Can you work these out from the model? Positions are in its coordinate system, mm. A direction names the side the tool comes from. Coordinates: 2 decimals unless noted, no trailing zeros. Order: outer loops, then holes, each group sorted by start corner. A loop starts at its lowest first (then second) coordinate and runs counter-clockwise, first axis right, second up. Notation, with made-up numbers: (-39, 30.25) - (16, 30.25) arc R22 cw to (16, 57.25) - close; hole circle Ø6 at (38, 74.5). An arc over 180 degrees is marked (long way). Return JSON: item names as keys, results as strings. Group by question number.
1) Which directions (+Z, -Z, +X, -X, +Y, -Y) give clear straight access to the entire face, cutting with the end or side of a thin tool? Please do faces 4 (the face through (2, -90.702, -6)), 5 (the face through (2, -103.702, -17)), 6 (the face through (1.97, -115.42, -86.6)).
2) For pin 1 Ø1 at (x, z) = (1, -129.5) entering from -Y; pin 2 Ø2 at (x, z) = (2.5, -23) entering from +Y; pin 3 Ø1.2 at (x, z) = (2.5, -37.5) entering from +Y, each with a flat end and sliding along its axis, tell me the tip position at first contact or that it passes through.
3) Imagine slicing it at A-A (y = -126). Write out the boundary of the cut face in (x, z) (3 decimals), and give its area (3 significant figures).
4) Imagine slicing it at D-D (y = -62.5). Write out the boundary of the cut face in (x, z).
5) If we mould it in two halves opening along Z, with no side actions, what happens to faces 1 (the face through (1.972, -92.206, 3.574)), 2 (the face through (2, -140.702, -33)), 3 (the face through (2, -130.702, -17))? For each: pulls with the +Z half, pulls with the -Z half, needs draft (parallel to the pull), parting line crosses it, or undercut.
6) Imagine slicing it at C-C (y = -113). Write out the boundary of the cut face in (x, z) (3 decimals), and give its area (3 significant figures).
7) If I drill on line 1 along Z through (x, y) = (2.2, -133) (3 decimals); line 2 along Z through (x, y) = (3.55, -105) (3 decimals); line 3 along Z through (x, y) = (3.1, -122) (3 decimals), over which ranges is the centre line in solid material (lowest first)?
```python
from build123d import *

# Parameters (mm, degrees)
SKETCH2_W           = 4
SKETCH2_H           = 27
BOSS_EXTRUDE1_DEPTH = 4
CUT_EXTRUDE1_DEPTH  = 10
BOSS_EXTRUDE2_DEPTH = 4


with BuildPart() as part:
    # Sketch2 → Boss-Extrude1 (new body)
    with BuildSketch(Plane(origin=(0, 0, 0), x_dir=(0, 0, -1), z_dir=(1, 0, 0))):
        with BuildLine():
            Line((53.344601804, -85.498776043), (74.987188297, -45.905868036))
            ThreePointArc((74.987188297, -45.905868036), (78.661054663, -42.101027368), (83.761812448, -40.70232204))
            Line((83.761812448, -40.70232204), (92.296503371, -40.70232204))
            Line((92.296503371, -40.70232204), (92.296503371, -44.70232204))
            Line((92.296503371, -44.70232204), (152.296503371, -44.70232204))
            Line((152.296503371, -44.70232204), (152.296503371, -40.70232204))
            Line((152.296503371, -40.70232204), (160.831194294, -40.70232204))
            ThreePointArc((160.831194294, -40.70232204), (165.931952079, -42.101027368), (169.605818445, -45.905868036))
            Line((169.605818445, -45.905868036), (191.248404938, -85.498776043))
            ThreePointArc((191.248404938, -85.498776043), (194.922271304, -89.303616711), (200.023029089, -90.70232204))
            Line((200.023029089, -90.70232204), (206.057918615, -90.70232204))
            Line((206.057918615, -90.70232204), (211.09280814, -90.70232204))
            Line((211.09280814, -90.70232204), (211.09280814, -94.70232204))
            Line((211.09280814, -94.70232204), (233.09280814, -94.70232204))
            Line((233.09280814, -94.70232204), (233.09280814, -90.70232204))
            Line((233.09280814, -90.70232204), (244.938223676, -90.70232204))
            ThreePointArc((244.938223676, -90.70232204), (248.5155042, -92.209033609), (249.936812742, -95.821096417))
            Line((249.936812742, -95.821096417), (248.986349517, -135.821096417))
            ThreePointArc((248.986349517, -135.821096417), (247.481048882, -139.279602563), (243.987760452, -140.70232204))
            Line((243.987760452, -140.70232204), (180.035244387, -140.70232204))
            ThreePointArc((180.035244387, -140.70232204), (175.292734587, -139.506218949), (171.684730912, -136.204042199))
            Line((171.684730912, -136.204042199), (144.669691073, -95.20060188))
            ThreePointArc((144.669691073, -95.20060188), (141.061687399, -91.89842513), (136.319177599, -90.70232204))
            Line((136.319177599, -90.70232204), (108.273829143, -90.70232204))
            ThreePointArc((108.273829143, -90.70232204), (103.531319343, -91.89842513), (99.923315669, -95.20060188))
            Line((99.923315669, -95.20060188), (72.90827583, -136.204042199))
            ThreePointArc((72.90827583, -136.204042199), (69.300272155, -139.506218949), (64.557762355, -140.70232204))
            Line((64.557762355, -140.70232204), (0, -140.70232204))
            ThreePointArc((0, -140.70232204), (-3.535533906, -139.237855945), (-5, -135.70232204))
            Line((-5, -135.70232204), (-5, -95.70232204))
            ThreePointArc((-5, -95.70232204), (-3.535533906, -92.166788134), (0, -90.70232204))
            Line((0, -90.70232204), (11.500198602, -90.70232204))
            Line((11.500198602, -90.70232204), (11.500198602, -94.70232204))
            Line((11.500198602, -94.70232204), (33.500198602, -94.70232204))
            Line((33.500198602, -94.70232204), (33.500198602, -90.70232204))
            Line((33.500198602, -90.70232204), (38.535088127, -90.70232204))
            Line((38.535088127, -90.70232204), (44.569977653, -90.70232204))
            ThreePointArc((44.569977653, -90.70232204), (49.670735438, -89.303616711), (53.344601804, -85.498776043))
        make_face()
        with Locations((227.463006742, -117.20232204)):
            Rectangle(SKETCH2_W, SKETCH2_H, mode=Mode.SUBTRACT)
        with Locations((17.13, -117.20232204)):
            Rectangle(SKETCH2_W, SKETCH2_H, mode=Mode.SUBTRACT)
    extrude(amount=BOSS_EXTRUDE1_DEPTH)

    # Sketch3 → Cut-Extrude1 (cut)
    with BuildSketch(Plane(origin=(0, 0, 0), x_dir=(0, 0, -1), z_dir=(1, 0, 0))):
        Polygon((160.831194294, -40.70232204), (160.831194294, -144.460869934), (257.875348239, -144.460869934), (257.875348239, -25.544082069), (160.831194294, -34.903829247), align=None)
    extrude(amount=CUT_EXTRUDE1_DEPTH, mode=Mode.SUBTRACT)

    # Sketch4 → Boss-Extrude2 (add)
    with BuildSketch(Plane(origin=(0, 0, 0), x_dir=(0, 0, -1), z_dir=(1, 0, 0))):
        with BuildLine():
            Line((160.831194294, -40.70232204), (180.831194294, -40.70232204))
            Line((180.831194294, -40.70232204), (180.831194294, -135.70232204))
            ThreePointArc((180.831194294, -135.70232204), (179.3667282, -139.237855945), (175.831194294, -140.70232204))
            Line((175.831194294, -140.70232204), (153.525004458, -140.70232204))
            ThreePointArc((153.525004458, -140.70232204), (149.989470552, -139.237855945), (148.525004458, -135.70232204))
            Line((148.525004458, -135.70232204), (148.525004458, -101.052198369))
            Line((148.525004458, -101.052198369), (160.831194294, -40.70232204))
        make_face()
    extrude(amount=BOSS_EXTRUDE2_DEPTH)


solid = part.part
```
Calculated:
{
 "1": {"face 4": "+Z, +X, -X, +Y", "face 5": "+X, -X", "face 6": "+X, -X, -Y"},
 "2": {"pin 1": "y = -90.7", "pin 2": "y = -94.7", "pin 3": "y = -90.7"},
 "3": {"outline": "(0, -180.831) - (4, -180.831) - (4, -148.525) - (0, -148.525) - close; (0, -79.631) - (4, -79.631) - (4, -19.13) - (0, -19.13) - close; (0, -15.13) - (4, -15.13) - (4, 5) - (0, 5) - close", "area": "452 mm2"},
 "4": {"outline": "(0, -180.83) - (4, -180.83) - (4, -65.92) - (0, -65.92) - close"},
 "5": {"face 1": "pulls with the +Z half", "face 2": "needs draft", "face 3": "undercut"},
 "6": {"outline": "(0, -180.831) - (4, -180.831) - (4, -148.525) - (0, -148.525) - close; (0, -88.196) - (4, -88.196) - (4, -19.13) - (0, -19.13) - close; (0, -15.13) - (4, -15.13) - (4, 5) - (0, 5) - close", "area": "486 mm2"},
 "7": {"line 1": "-180.831 to -148.525, -75.019 to 5", "line 2": "-180.831 to -148.525, -93.467 to -19.13, -15.13 to 5", "line 3": "-180.831 to -148.525, -82.267 to -19.13, -15.13 to 5"}
}
